```python
from build123d import *

# Parameters (mm, degrees)
SKETCH1_R       = 2
EXTRUDE1_DEPTH  = 10
EXTRUDE2_DEPTH  = 8
SKETCH3_R       = 4
EXTRUDE3_DEPTH  = 6.5
SKETCH19_R      = 1.5
EXTRUDE13_DEPTH = 51
FILLET11_R      = 1


with BuildPart() as part:
    # Sketch1 → Extrude1 (new body)
    with BuildSketch(Plane.XY):
        Circle(SKETCH1_R)
    extrude(amount=-EXTRUDE1_DEPTH)

    # Sketch2 → Extrude2 (cut)
    with BuildSketch(Plane.XY):
        with BuildLine():
            Line((-1.322875656, 1.5), (1.322875656, 1.5))
            ThreePointArc((1.322875656, 1.5), (0, 2), (-1.322875656, 1.5))
        make_face()
    extrude(amount=-EXTRUDE2_DEPTH, mode=Mode.SUBTRACT)

    # Sketch3 → Extrude3 (add)
    with BuildSketch(Plane(origin=(0, 0, -10), x_dir=(-1, 0, 0), z_dir=(0, 0, -1))):
        Circle(SKETCH3_R)
    extrude(amount=EXTRUDE3_DEPTH)

    # Sketch19 → Extrude13 (add)
    with BuildSketch(Plane(origin=(0, 0, -16.5), x_dir=(-1, 0, 0), z_dir=(0, 0, -1))):
        Circle(SKETCH19_R)
    extrude(amount=EXTRUDE13_DEPTH)

    # Fillet11
    fillet11_edges = [part.edges().sort_by_distance(p)[0] for p in [
        (1.5, 0, -67.5),
    ]]
    fillet(fillet11_edges, radius=FILLET11_R)


solid = part.part
```
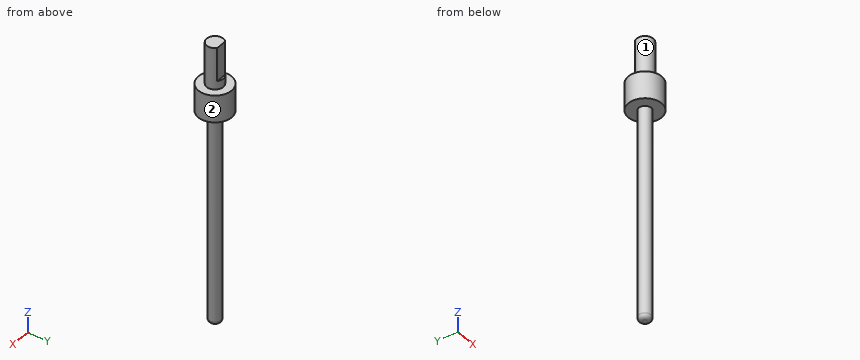
Check sheet for the modelled part. Datum: model origin and axes. Units: mm. Face numbers are marked on the shaded views. A direction names the side the tool comes from. Give positions to 0.01 mm unless a question says otherwise; leave off trailing zeros. Write each loop counter-clockwise with the first axis right and the second up, starting at its lowest first coordinate (ties: lowest second). Pieces come first, ordered by that corner, then holes.
Item 1: Cross-section at D-D (z = -32). Enter the section's corners in (x, y).
Item 2: Cross-section at A-A (z = -12.5). Enter the section's corners in (x, y), and give its area (3 significant figures).
Item 3: Cross-section at B-B (x = 3). Enter the section's corners in (y, z), and give its area (3 significant figures).
Item 4: Gauge pin test, flat ends, axial feed: pin 1 (3 mm diameter, centred on x = -2.5, y = 2, fed in from -Z); pin 2 (1 mm diameter, centred on x = 2.5, y = 0.5, fed in from +Z); pin 3 (1.5 mm diameter, centred on x = 0.5, z = -29.5, fed in from -Y). Record the tip position at first contact, or that the pin passes through.
Item 5: Access from +Z, -Z, +X, -X, +Y, -Y to the whole of each face (thin tool, end or side, straight path). Record for the marked faces 1 and 2.
Item 6: Scan lines: L1, parallel to Y at x = -0.25, z = -15.5; L2, parallel to Z at x = 1.5, y = -1.5; L3, parallel to Y at x = 0, z = -21.5. Record each from-to range of solid material in increasing order.
Report:
1. outline: circle Ø3 at (0, 0)
2. outline: circle Ø8 at (0, 0)
2. area: 50.3 mm2
3. outline: (-2.65, -16.5) - (2.65, -16.5) - (2.65, -10) - (-2.65, -10) - close
3. area: 34.4 mm2
4. pin 1: stops at z = -16.5
4. pin 2: stops at z = -10
4. pin 3: stops at y = -1.5
5. face 1: +Z
5. face 2: +Z, -Z
6. L1: y = -3.99 to 3.99
6. L2: z = -16.5 to -10
6. L3: y = -1.5 to 1.5
